```python
from build123d import *

# Parameters (mm, degrees)
F1_DEPTH = 44
F3_DEPTH = 79
F4_R     = 5


with BuildPart() as f1:
    # F0 (on Top) → F1 (new body)
    with BuildSketch(Plane.XY):
        with BuildLine():
            Line((35, 85), (35, 0))
            Line((35, 0), (39, 0))
            ThreePointArc((39, 0), (92.033008589, 21.966991411), (114, 75))
            Line((114, 75), (114, 595))
            Line((114, 595), (35, 595))
            Line((35, 595), (35, 745))
            Line((35, 745), (15, 745))
            Line((15, 745), (15, 740))
            Line((15, 740), (0, 725))
            Line((0, 725), (0, 105))
            Line((0, 105), (15, 90))
            Line((15, 90), (15, 85))
            Line((15, 85), (35, 85))
        make_face()
    extrude(amount=-F1_DEPTH)

    # F2 (on face) → F3 (cut)
    with BuildSketch(Plane.YZ.offset(114)):
        Polygon((595, -44), (595, 0), (583.210235533, -44), align=None)
    extrude(amount=-F3_DEPTH, mode=Mode.SUBTRACT)

    # F4
    f4_edges = [f1.edges().sort_by_distance(p)[0] for p in [
        (37, 0, 0),
        (114, 329.105118, -44),
        (0, 415, 0),
        (0, 415, -44),
        (74.5, 595, 0),
    ]]
    fillet(f4_edges, radius=F4_R)


solid = f1.part
```
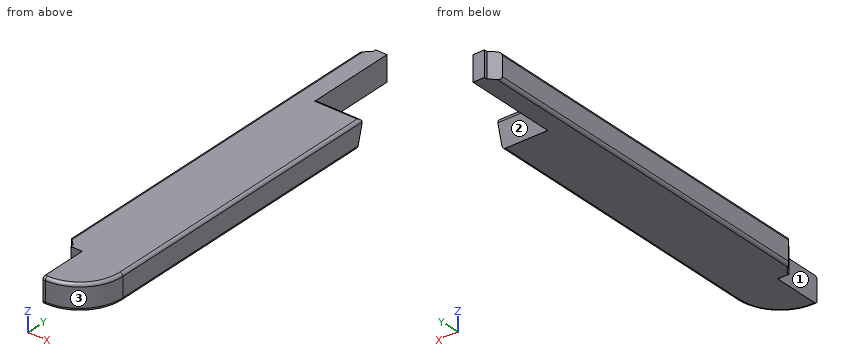
Can you work these out from the model? Positions are in its coordinate system, mm. Face numbers are marked on the shaded views. A direction names the side the tool comes from. Round coordinates to 2 decimals unless told otherwise and drop trailing zeros. Order: outer loops, then holes, each group sorted by start corner. A loop starts at its lowest first (then second) coordinate and runs counter-clockwise, first axis right, second up. Notation, with made-up numbers: (7, 73.25) -> (18, 73.25) arc R31 cw to (18, 109.25) -> close; hole circle Ø3 at (-22.75, -29.75). An arc over 180 degrees is marked (long way). Return JSON: item names as keys, results as strings. Group by question number.
1. If we section it at A-A, the plane z = -31.5: Write out the boundary of the cut face in (x, y), then the cut area to 3 significant figures.
2. If we section it at B-B, the plane y = 694: Write out the boundary of the cut face in (x, z).
3. I need wall thicknesses on line 1 (X direction, y = 217, z = -39.5); line 2 (X direction, y = 614, z = -22); line 3 (Y direction, x = 25, z = -35). Which ranges of each line are inside material? Lowest first, please. Write a range as [from, to].
4. Will these pins go through, and if not, where does the flat tip stop? pin 1 (2.5 mm diameter, centred on y = 87.5, z = -12.5, fed in from -X); pin 2 (12 mm diameter, centred on y = 646, z = -4.5, fed in from +X); pin 3 (5.5 mm diameter, centred on y = 742, z = -29, fed in from -X).
5. If we section it at C-C, the plane x = 22.5: Write out the boundary of the cut face in (y, z), then the cut area to 3 significant figures.
6. Which directions (+Z, -Z, +X, -X, +Y, -Y) give clear straight access to the entire face, cutting with the end or side of a thin tool? Please do the marked faces 1, 2 and 3.
Output values:
{
 "1": {"outline": "(0, 105) -> (15, 90) -> (15, 85) -> (35, 85) -> (35, 0) -> (39, 0) arc R75 ccw to (114, 75) -> (114, 586.56) -> (35, 586.56) -> (35, 745) -> (15, 745) -> (15, 740) -> (0, 725) -> close", "area": "67,900 mm²"},
 "2": {"outline": "(0, -39) arc R5 ccw to (5, -44) -> (35, -44) -> (35, 0) -> (5, 0) arc R5 ccw to (0, -5) -> close"},
 "3": {"line 1": "[0.03, 113.97]", "line 2": "[0, 35]", "line 3": "[85, 745]"},
 "4": {"pin 1": "x = 15", "pin 2": "x = 35", "pin 3": "x = 14.25"},
 "5": {"outline": "(85, -44) -> (745, -44) -> (745, 0) -> (85, 0) -> close", "area": "29,000 mm²"},
 "6": {"face 1": "+Z, -Z, -X, -Y", "face 2": "-Z, +X, +Y", "face 3": "+Z, -Z, +X, -Y"}
}
